```python
from build123d import *

# Parameters (mm, degrees)
BOSS_EXTRUDE2_DEPTH     = 15
SKETCH4_R               = 10.25
CUT_EXTRUDE1_DEPTH      = 39
SKETCH5_R               = 1
CUT_EXTRUDE2_DEPTH      = 46
CUT_EXTRUDE4_DEPTH      = 30
CUT_EXTRUDE4_DEPTH_BACK = 20
SKETCH8_W               = 87.305200023
SKETCH8_H               = 11.791688203
SKETCH9_R               = 1.5
CUT_EXTRUDE5_DEPTH      = 45


with BuildPart() as part:
    # Sketch2 → Boss-Extrude2 (new body)
    with BuildSketch(Plane.XY):
        with BuildLine():
            Line((29.39514737, -26.166473039), (19.28603361, -26.166473039))
            ThreePointArc((19.28603361, -26.166473039), (14.916401147, -24.5745939), (12.952232935, -20.359168619))
            ThreePointArc((12.952232935, -20.359168619), (-3.527212702, -8.286066454), (-6.642968051, 11.903633717))
            Line((-6.642968051, 11.903633717), (-6.642968051, 13.194145811))
            ThreePointArc((-6.642968051, 13.194145811), (-12.734188373, 17.984078311), (-13.654337816, 25.678215258))
            ThreePointArc((-13.654337816, 25.678215258), (-5.75878812, 24.441537952), (-1.050254298, 17.984078311))
            ThreePointArc((-1.050254298, 17.984078311), (12.191739255, 21.923154941), (24.34059049, 15.3449993))
            ThreePointArc((24.34059049, 15.3449993), (36.489441725, 21.923154941), (49.731435279, 17.984078311))
            ThreePointArc((49.731435279, 17.984078311), (54.439969101, 24.441537952), (62.335518797, 25.678215258))
            ThreePointArc((62.335518797, 25.678215258), (61.415369354, 17.984078311), (55.324149032, 13.194145811))
            Line((55.324149032, 13.194145811), (55.324149032, 11.903633717))
            ThreePointArc((55.324149032, 11.903633717), (52.208393682, -8.286066454), (35.728948045, -20.359168619))
            ThreePointArc((35.728948045, -20.359168619), (33.764779834, -24.5745939), (29.39514737, -26.166473039))
        make_face()
    extrude(amount=BOSS_EXTRUDE2_DEPTH)

    # Sketch4 → Cut-Extrude1 (cut)
    with BuildSketch(Plane.XY):
        with Locations((12.237485625, 0)):
            Circle(SKETCH4_R)
        with Locations((38.237485625, 1.902154712)):
            Circle(SKETCH4_R)
        with BuildLine():
            Line((18.291353785, -14.692373008), (30.14458787, -14.692373008))
            ThreePointArc((30.14458787, -14.692373008), (24.217970827, -17.965213498), (18.291353785, -14.692373008))
        make_face()
    extrude(amount=CUT_EXTRUDE1_DEPTH, mode=Mode.SUBTRACT)

    # Sketch5 → Cut-Extrude2 (cut)
    with BuildSketch(Plane.XY):
        with Locations((3.966291552, -9.460600721)):
            Circle(SKETCH5_R)
        with Locations((45.466291552, -8.281636769)):
            Circle(SKETCH5_R)
    extrude(amount=CUT_EXTRUDE2_DEPTH, mode=Mode.SUBTRACT)

    # Sketch8 → Cut-Extrude4 (cut, two sides: drawn at the far end of the back side and taken through both)
    with BuildSketch(Plane(origin=(0, 0, 0), x_dir=(1, 0, 0), z_dir=(0, 1, 0)).offset(-CUT_EXTRUDE4_DEPTH_BACK)):
        with Locations((24.422336933, -5.895844102)):
            Rectangle(SKETCH8_W, SKETCH8_H)
    extrude(amount=CUT_EXTRUDE4_DEPTH + CUT_EXTRUDE4_DEPTH_BACK, mode=Mode.SUBTRACT)

    # Sketch9 → Cut-Extrude5 (cut)
    with BuildSketch(Plane(origin=(0, 0, 0), x_dir=(1, 0, 0), z_dir=(0, 1, 0))):
        with Locations(Location((24.831069142, -5.82419794, 0), (0, 0, 270))):
            Circle(SKETCH9_R)
    extrude(amount=-CUT_EXTRUDE5_DEPTH, mode=Mode.SUBTRACT)


solid = part.part
```
Geometry check sheet. Reference: the model listing, model coordinates, mm. A direction names the side the tool comes from. Round coordinates to 2 decimals unless told otherwise and drop trailing zeros. Loops run counter-clockwise (first coordinate to the right, second up) from the corner with the lowest first, then second, coordinate; pieces in that order, holes last. Notation, with made-up numbers: M -38.5,58 L -27.5,58 A26 ccw -27.5,74 Z; hole C 31,68 d11. An arc over 180 degrees is marked long. Return JSON: item names as keys, results as strings. Group by question number.
(1) Set-up check for faces 4 (the face through (24, -20, 8)), 5 (the face through (24, -14.692, 13)), 6 (the face through (-12.68, 17.89, 13.37)): record each of +Z, -Z, +X, -X, +Y, -Y from which the full face is reachable in a straight line by a thin tool's end or side.
(2) Scan lines: line 1 along X through (y, z) = (8, 12.25); line 2 along X through (y, z) = (0, 13.9); line 3 along X through (y, z) = (-20.5, 9.25). Record each from-to range of solid material in increasing order. Write a range as [from, to].
(3) Section check D-D, the plane y = 0. Enter the section's corners in (x, z), and give its area (3 significant figures).
(4) Mould release check, pull along Y, two halves, no side actions. Record for faces 1 (the face through (14.966, -24.619, 7.395)), 2 (the face through (11.994, 21.943, 13.373)), 3 (the face through (24.317, -17.965, 13.373)): pulls with the +Y half, pulls with the -Y half, needs draft (parallel to the pull), parting line crosses it, or undercut.
(5) Section check C-C, the plane z = 12.75. Give the number of separate pieces and of enclosed holes in the cut face, and give its area (3 significant figures).
(6) Section check A-A, the plane y = 17. Enter the section's corners in (x, z).
(7) Section check B-B, the plane z = 9. Enter the section's corners in (x, y).
(8) Go/stop test with flat-tipped pins: pin 1 (6 mm diameter, centred on x = 43, z = 11.5, fed in from -Y); pin 2 (3 mm diameter, centred on x = 26.5, z = 4, fed in from -Y); pin 3 (1 mm diameter, centred on y = 12.5, z = 13.5, fed in from -X). Record where each tip stops, or that it passes through.
Data:
{
 "1": {"face 4": "-Z, +X, -X, +Y", "face 5": "+Z, -Z", "face 6": "+Z, -Z, -X"},
 "2": {"line 1": "[-7.29, 5.83], [18.65, 30], [46.48, 55.98]", "line 2": "[-6.82, 1.99], [22.49, 28.17], [48.31, 55.5]", "line 3": "[12.96, 35.72]"},
 "3": {"outline": "M -6.82,11.79 L 1.99,11.79 L 1.99,15 L -6.82,15 Z; M 22.49,11.79 L 28.17,11.79 L 28.17,15 L 22.49,15 Z; M 48.31,11.79 L 55.5,11.79 L 55.5,15 L 48.31,15 Z", "area": "69.5 mm²"},
 "4": {"face 1": "pulls with the -Y half", "face 2": "pulls with the +Y half", "face 3": "undercut"},
 "5": {"separate pieces": "1", "enclosed holes": "5", "area": "1,890 mm²"},
 "6": {"outline": "M -12.1,11.79 L 22.82,11.79 L 22.82,15 L -12.1,15 Z; M 25.86,11.79 L 60.79,11.79 L 60.79,15 L 25.86,15 Z"},
 "7": {"outline": "M 11.63,-20 A26.69 ccw 12.95,-20.36 A6.08 ccw 19.29,-26.17 L 29.4,-26.17 A6.08 ccw 35.73,-20.36 A26.69 ccw 37.05,-20 Z"},
 "8": {"pin 1": "y = -18.92", "pin 2": "y = -26.17", "pin 3": "x = -6.64"}
}
